The model under review builds one solid part; all positions refer to its coordinate system, in mm. A direction names the side the tool comes from. Give positions to 0.01 mm unless a question says otherwise; leave off trailing zeros. Loops run counter-clockwise (first coordinate to the right, second up) from the corner with the lowest first, then second, coordinate; pieces in that order, holes last. Notation, with made-up numbers: M -19,63.25 L -1,63.25 A30 cw -1,95.25 Z; hole C -24,22 d5. An arc over 180 degrees is marked long. Put each result on its own line as item: value. Start each with the question number.
from build123d import *

# Parameters (mm, degrees)
CHAFL_N1_SIZE = 0.45
CHAFL_N2_SIZE = 0.5


with BuildPart() as part:
    # Croquis1 → Revolución1 (revolve)
    with BuildSketch(Plane(origin=(0, 0, 0), x_dir=(0, 0, -1), z_dir=(1, 0, 0))):
        with BuildLine():
            Line((0, 0), (0, 5))
            Line((0, 5), (18, 5))
            Line((18, 5), (18, 35.5))
            Line((18, 35.5), (25, 35.5))
            Line((25, 35.5), (25, 5))
            ThreePointArc((25, 5), (25.8, 4.2), (26.6, 5))
            Line((26.6, 5), (33, 5))
            Line((33, 5), (40.464101615, 3))
            Line((40.464101615, 3), (49.464101615, 3))
            Line((49.464101615, 3), (49.464101615, 0))
            Line((49.464101615, 0), (0, 0))
        make_face()
    revolve(axis=Axis((0, 0, -49.464101615), (0, 0, 1)))

    # Chaflán1
    chafl_n1_edges = [part.edges().sort_by_distance(p)[0] for p in [
        (0, -3, -49.464101615),
    ]]
    chamfer(chafl_n1_edges, length=CHAFL_N1_SIZE)

    # Chaflán2
    chafl_n2_edges = [part.edges().sort_by_distance(p)[0] for p in [
        (0, -5, 0),
    ]]
    chamfer(chafl_n2_edges, length=CHAFL_N2_SIZE)


solid = part.part
(1) Insertion check: pin 1 (3 mm diameter, centred on x = -21.5, y = 18, fed in from +Z); pin 2 (6 mm diameter, centred on x = -16.5, z = -24.5, fed in from -Y); pin 3 (8 mm diameter, centred on y = -15, z = -26, fed in from +X); pin 4 (21.5 mm diameter, centred on x = -0.5, y = -9.5, fed in from +Z). Each pin has a flat end and moves straight along its axis. Give the tip position at first contact, or say it passes through.
(2) We need section A-A, the plane x = 0. Write out the cut boundary in (y, z).
(3) We need section D-D, the plane z = -19.5. Write out the cut boundary in (x, y).
(4) We need section C-C, the plane z = -8. Write out the cut boundary in (x, y), plus the area to 3 significant figures.
(5) For faces 1 (the cylindrical face through (4.88, -1.08, -9.37)), 2 (the cylindrical face through (0, -3, -45)), 3 (the flat face through (0, 0, -49.464)), list the 3-axis set-ups (+Z, -Z, +X, -X, +Y, -Y) from which the entire face can be reached by the end or side of a thin tool; tool diameter is ignored.
(6) To check wall thickness, follow L1, parallel to Z at x = 27, y = -9; L2, parallel to X at y = -0.5, z = -19.5; L3, parallel to X at y = 28, z = -22. State the ranges of each line that lie inside material, in increasing order. Write a range as [from, to].
Check sheet entries:
1. pin 1: stops at z = -18
1. pin 2: stops at y = -32.83
1. pin 3: stops at x = 33.71
1. pin 4: stops at z = 0
2. outline: M -35.5,-25 L -5,-25 A0.8 cw -5,-26.6 L -5,-33 L -3,-40.46 L -3,-49.01 L -2.55,-49.46 L 2.55,-49.46 L 3,-49.01 L 3,-40.46 L 5,-33 L 5,-26.6 A0.8 cw 5,-25 L 35.5,-25 L 35.5,-18 L 5,-18 L 5,-0.5 L 4.5,0 L -4.5,0 L -5,-0.5 L -5,-18 L -35.5,-18 Z
3. outline: C 0,0 d71
4. outline: C 0,0 d10
4. area: 78.5 mm²
5. face 1: +Z
5. face 2: -Z
5. face 3: -Z, +X, -X, +Y, -Y
6. L1: z = [-25, -18]
6. L2: x = [-35.5, 35.5]
6. L3: x = [-21.82, 21.82]
